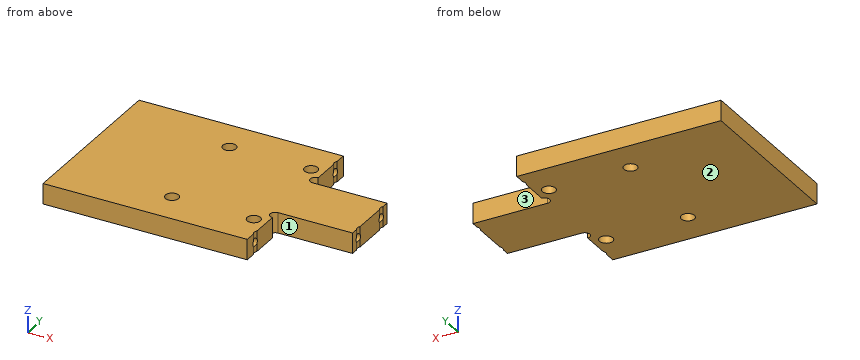
Autodesk Inventor part; units mm, degrees
ref_plane "YZ Plane" through (0, 0, 0) normal (1, 0, 0) x (0, 1, 0)
ref_plane "XZ Plane" through (0, 0, 0) normal (0, 1, 0) x (-1, 0, 0)
ref_plane "XY Plane" through (0, 0, 0) normal (0, 0, 1) x (1, 0, 0)
sketch "スケッチ1" plane through (0, 0, 0) normal (0, 0, 1) x (1, 0, 0)
  line L0 (14, 10) -> (30, 10) construction
  line L1 (30, 10) -> (30, -10) construction
  line L2 (30, -10) -> (14, -10) construction
  line L3 (14, -10) -> (14, 10) construction
  line L4 (0, 0) -> (42.5052, 0) construction
  line L5 (-7.5, 16.75) -> (32.5, 16.75)
  line L6 (47.1, 6) -> (47.1, 4.6)
  line L7 (32.5, -16.75) -> (-7.5, -16.75)
  line L8 (32.5, 16.75) -> (32.5, 14.6)
  line L9 (32.5, 8) -> (32.5, 6) construction
  line L10 (32.5, 6) -> (47.1, 6)
  arc A0 (32.5, 8) -> (32.5, 6) centre (32.5, 7) ccw
  line L11 (32.5, -16.75) -> (32.5, -14.6)
  line L12 (32.5, -6) -> (47.1, -6)
  arc A1 (32.5, -6) -> (32.5, -8) centre (32.5, -7) ccw
  line L13 (32.5, 6) -> (32.5, -6) construction
  line L14 (32.5, -8) -> (32.5, -6) construction
  arc A2 (47.1, 4.6) -> (47.1, 3.4) centre (47.9, 4) ccw
  arc A3 (47.1, -3.4) -> (47.1, -4.6) centre (47.9, -4) ccw
  line L15 (47.1, 4.6) -> (47.1, 3.4) construction
  line L16 (47.1, 3.4) -> (47.1, -3.4)
  line L17 (47.1, -3.4) -> (47.1, -4.6) construction
  line L18 (47.1, -4.6) -> (47.1, -6)
  arc A4 (32.5, 14.6) -> (32.5, 13.4) centre (33.3, 14) ccw
  line L19 (32.5, 13.4) -> (32.5, 8)
  line L20 (32.5, 14.6) -> (32.5, 13.4) construction
  line L21 (33.7, 6) -> (33.7, -6) construction
  arc A5 (32.5, -13.4) -> (32.5, -14.6) centre (33.3, -14) ccw
  line L22 (32.5, -13.4) -> (32.5, -8)
  line L23 (32.5, -14.6) -> (32.5, -13.4) construction
  line L24 (-7.5, 16.75) -> (-7.5, -16.75)
  line L25 (35.7, 6) -> (35.7, -6) construction
  dimension "d0" = 20
  dimension "d1" = 16
  dimension "d3" = 1
  dimension "d4" = 12
  dimension "d5" = 2.5
  dimension "d7" = 1
  dimension "d8" = 0.8
  dimension "d9" = 8
  dimension "d10" = 0.8
  dimension "d11" = 28
  dimension "d12" = 33.5
  dimension "d29" = 1.2
  dimension "d32" = 40
  dimension "d34" = 32.5
  dimension "d36" = 2
  dimension "d37" = 11.4
extrude "押し出し1" add sketch "スケッチ1" along normal blind 4
hole "穴1" at (14, 10, 0) at (30, 10, 0) at (30, -10, 0) at (14, -10, 0) direction (0, 0, 1) diameter 2.6 end through all
sketch "スケッチ2" plane through (32.5, 8, 0) normal (1, 0, 0) x (0, 0, -1)
  line L0 (0, 6.6) -> (-4, 6.6) construction
  line L1 (0, 5.4) -> (-4, 5.4) construction
  line L2 (-4, 6.6) -> (0, 5.4) construction
  line L3 (0, -21.4) -> (-4, -21.4) construction
  line L4 (0, -22.6) -> (-4, -22.6) construction
  line L5 (-4, -21.4) -> (0, -22.6) construction
  point P0 (0, -8)
  point P1 (-2, 6)
  point P2 (-2, -22)
hole "穴2" at (32.5, 14, 2) at (32.5, -14, 2) direction (-1, 0, 0) diameter 1.567 depth 6 tip angle 118
sketch "スケッチ3" plane through (47.1, -3.4, 0) normal (1, 0, 0) x (0, 0, -1)
  line L0 (0, -1.2) -> (-4, -1.2) construction
  line L1 (0, 0) -> (-4, 0) construction
  line L2 (0, -1.2) -> (-4, 0) construction
  line L3 (0, 6.8) -> (-4, 6.8) construction
  line L4 (0, 8) -> (-4, 8) construction
  line L5 (0, 6.8) -> (-4, 8) construction
  point P0 (0, 3.4)
  point P1 (-2, -0.6)
  point P2 (-2, 7.4)
hole "穴3" at (47.1, -4, 2) at (47.1, 4, 2) direction (-1, 0, 0) diameter 1.567 depth 6.3 tip angle 118
properties part number "SERVO_MOUNT_TIP"
The listing builds one solid part. Answer for the finished solid, in the listing's coordinates (mm). Face numbers are marked on the shaded views. A direction names the side the tool comes from. Round coordinates to 2 decimals unless told otherwise and drop trailing zeros. Write each loop counter-clockwise with the first axis right and the second up, starting at its lowest first coordinate (ties: lowest second). Pieces come first, ordered by that corner, then holes. Notation, with made-up numbers: (-4.75, 3.25) - (30.25, 3.25) arc R31 cw to (30.25, 35.25) - close; hole circle Ø9 at (29.25, 24.5). An arc over 180 degrees is marked (long way). Use a Markdown table: item, result. Add a question column.
1. The part is cut by section A-A (x = 30). Write down the section's boundary in (y, z), and give its area (3 significant figures).
2. A tool of negligible diameter and unlimited length cuts with its end or side. For the marked faces 1, 2 and 3, from which of +Z, -Z, +X, -X, +Y, -Y can it reach the whole face along a straight path? Write none if from no direction.
3. Consider line 1 (Y direction, x = 45, z = 2); line 2 (X direction, y = 10, z = 2.7); line 3 (Y direction, x = 14, z = 1). Determine where each line is inside the solid, lowest interval first.
4. The part is cut by section B-B (y = -10). Write down the section's boundary in (x, z).
5. Flat-ended cylindrical pins translate along their axes: P1, Ø0.9, axis at y = -14, z = 2, coming from the +X side; P2, Ø1.7, axis at y = -16, z = 2, coming from the +X side; P3, Ø1.3, axis at y = 14, z = 2, coming from the +X side; P4, Ø2, axis at x = 30, y = 10, coming from the +Z side. Find the tip coordinate at first contact, or state that the pin passes through.
Reported:
| question | item | result |
|---|---|---|
| 1 | outline | (-16.75, 0) - (-11.3, 0) - (-11.3, 4) - (-16.75, 4) - close; (-8.7, 0) - (8.7, 0) - (8.7, 4) - (-8.7, 4) - close; (11.3, 0) - (16.75, 0) - (16.75, 4) - (11.3, 4) - close; hole circle Ø1.57 at (-14, 2); hole circle Ø1.57 at (14, 2) |
| 1 | area | 109 mm^2 |
| 2 | face 1 | +Z, -Z, +X, -Y |
| 2 | face 2 | -Z, +X, -X, +Y, -Y |
| 2 | face 3 | +Z, -Z, +X, +Y |
| 3 | line 1 | -6 to -4.78, -3.22 to 3.22, 4.78 to 6 |
| 3 | line 2 | -7.5 to 12.7, 15.3 to 28.7, 31.3 to 32.5 |
| 3 | line 3 | -16.75 to -11.3, -8.7 to 8.7, 11.3 to 16.75 |
| 4 | outline | (-7.5, 0) - (12.7, 0) - (12.7, 4) - (-7.5, 4) - close; (15.3, 0) - (28.7, 0) - (28.7, 4) - (15.3, 4) - close; (31.3, 0) - (32.5, 0) - (32.5, 4) - (31.3, 4) - close |
| 5 | P1 | x = 26.3 |
| 5 | P2 | x = 32.5 |
| 5 | P3 | x = 26.42 |
| 5 | P4 | through |
